Work out the finished part from the listing and answer in its coordinate system (mm). Give positions to 0.01 mm unless a question says otherwise; leave off trailing zeros. Write each loop counter-clockwise with the first axis right and the second up, starting at its lowest first coordinate (ties: lowest second). Pieces come first, ordered by that corner, then holes. Notation, with made-up numbers: (88.5, 53) - (117.5, 53) arc R15 ccw to (117.5, 70) - close; hole circle Ø7 at (-38.75, -14). An arc over 180 degrees is marked (long way). Write item = value, one per line.
Autodesk Inventor part; units mm, degrees
ref_plane "YZ Plane" through (0, 0, 0) normal (1, 0, 0) x (0, 1, 0)
ref_plane "XZ Plane" through (0, 0, 0) normal (0, 1, 0) x (-1, 0, 0)
ref_plane "XY Plane" through (0, 0, 0) normal (0, 0, 1) x (1, 0, 0)
sketch "Sketch1" plane through (0, 0, 0) normal (0, 1, 0) x (-1, 0, 0)
  line L0 (0, 0) -> (32.15, 0)
  line L1 (32.15, 0) -> (32.15, -32.15)
  line L2 (32.15, -32.15) -> (0, -32.15)
  line L3 (0, -32.15) -> (0, 0)
  circle A0 centre (29.0575, -5.89) radius 1.75
  circle A1 centre (29.0575, -26.26) radius 1.75
  line L4 (32.15, -16.075) -> (0, -16.075) construction
  line L5 (29.0575, -5.89) -> (3.0925, -5.89) construction
  line L6 (3.0925, -5.89) -> (3.0925, -26.26) construction
  line L7 (3.0925, -26.26) -> (29.0575, -26.26) construction
  line L8 (29.0575, -26.26) -> (29.0575, -5.89) construction
  circle A2 centre (3.0925, -5.89) radius 1.75
  circle A3 centre (3.0925, -26.26) radius 1.75
  line L9 (29.0575, -5.89) -> (3.0925, -26.26) construction
  circle A4 centre (24.965, -28.075) radius 0.635
  circle A5 centre (22.425, -28.075) radius 0.635
  circle A6 centre (19.885, -28.075) radius 0.635
  circle A7 centre (17.345, -28.075) radius 0.635
  circle A8 centre (14.805, -28.075) radius 0.635
  circle A9 centre (12.265, -28.075) radius 0.635
  circle A10 centre (9.725, -28.075) radius 0.635
  circle A11 centre (7.185, -28.075) radius 0.635
  circle A12 centre (24.965, -4.075) radius 0.635
  circle A13 centre (22.425, -4.075) radius 0.635
  circle A14 centre (19.885, -4.075) radius 0.635
  circle A15 centre (17.345, -4.075) radius 0.635
  circle A16 centre (14.805, -4.075) radius 0.635
  circle A17 centre (12.265, -4.075) radius 0.635
  circle A18 centre (9.725, -4.075) radius 0.635
  circle A19 centre (7.185, -4.075) radius 0.635
  line L10 (24.965, -4.075) -> (7.185, -28.075) construction
  circle A20 centre (30.9625, -21.155) radius 0.635
  circle A21 centre (30.9625, -18.615) radius 0.635
  circle A22 centre (30.9625, -16.075) radius 0.635
  circle A23 centre (30.9625, -13.535) radius 0.635
  circle A24 centre (30.9625, -10.995) radius 0.635
  circle A25 centre (1.1875, -21.155) radius 0.635
  circle A26 centre (1.1875, -18.615) radius 0.635
  circle A27 centre (1.1875, -16.075) radius 0.635
  circle A28 centre (1.1875, -13.535) radius 0.635
  circle A29 centre (1.1875, -10.995) radius 0.635
  line L11 (30.9625, -21.155) -> (1.1875, -10.995) construction
  point P0 (29.0575, -16.075)
  point P1 (16.075, -16.075)
  dimension "d0" = 32.15
  dimension "d1" = 32.15
  dimension "d3" = 20.37
  dimension "d4" = 3.5
  dimension "d5" = 3.5
  dimension "d6" = 3.5
  dimension "d7" = 3.5
  dimension "d8" = 25.965
  dimension "d9" = 1.27
  dimension "d12" = 2.54
  dimension "d15" = 24
  dimension "d20" = 1.27
  dimension "d23" = 2.54
  dimension "d26" = 29.775
extrude "Extrusion1" add sketch "Sketch1" along normal blind 1.6
equation "\"d5\" = d4"
equation "\"d6\" = d4"
equation "\"d7\" = d4"
equation "\"d20\" = d9"
properties part number "PCB"
1. Find section C-C, the plane y = 1. Give the number of separate pieces and of enclosed holes in the cut face, then the cut area to 3 significant figures.
Solution:
separate_pieces = 1
enclosed_holes = 30
area = 962 mm^2
2. Find section B-B, the plane x = -12. Give the vertices of the cut face in (y, z), then the cut area to 3 significant figures.
Solution:
outline = (0, -32.15) - (1.6, -32.15) - (1.6, -28.65) - (0, -28.65) - close; (0, -27.5) - (1.6, -27.5) - (1.6, -4.65) - (0, -4.65) - close; (0, -3.5) - (1.6, -3.5) - (1.6, 0) - (0, 0) - close
area = 47.7 mm^2
3. Straight lines are drawn through the part: line 1 (Z direction, x = -3, y = 1.25); line 2 (Z direction, x = -20, y = 0.3); line 3 (X direction, y = 1.2, z = -14). For each, find the intervals that lie inside material, in ascending order.
Solution:
line_1 = -32.15 to -28.01, -24.51 to -7.64, -4.14 to 0
line_2 = -32.15 to -28.7, -27.45 to -4.7, -3.45 to 0
line_3 = -32.15 to -31.39, -30.53 to -1.62, -0.76 to 0
4. For a pull along X with two mould halves and no side action, classify faces 1 (the cylindrical face through (-12.182, 0.789, -28.705)), 2 (the cylindrical face through (-1.105, 0.789, -21.785)), 3 (the flat face through (-16, 1, 0)) as pulls with the +X half, pulls with the -X half, needs draft (parallel to the pull), parting line crosses it, or undercut.
Solution:
face_1 = undercut
face_2 = undercut
face_3 = needs draft
5. Given pin 1 (2 mm diameter, centred on x = -3.09, z = -5.89, fed in from +Y), flat-ended and moving along its own axis, determine where the tip first touches the part or whether it passes through.
Solution:
pin_1 = through
6. Find section A-A, the plane z = -5.89. Give the vertices of the cut face in (x, y), then the cut area to 3 significant figures.
Solution:
outline = (-32.15, 0) - (-30.81, 0) - (-30.81, 1.6) - (-32.15, 1.6) - close; (-27.31, 0) - (-4.84, 0) - (-4.84, 1.6) - (-27.31, 1.6) - close; (-1.34, 0) - (0, 0) - (0, 1.6) - (-1.34, 1.6) - close
area = 40.2 mm^2
